Could you check a few things on this model? Use its own coordinates, in mm. Face numbers are marked on the shaded views. Coordinates: 2 decimals unless noted, no trailing zeros. Loops run counter-clockwise (first coordinate to the right, second up) from the corner with the lowest first, then second, coordinate; pieces in that order, holes last.
from build123d import *

# Parameters (mm, degrees)
GEARBOX_MOUNT_DEPTH  = 77
BOSS_EXTRUDE6_START  = 38
SKETCH7_R            = 1.7
SKETCH7_W            = 1
SKETCH7_H            = 6
BOSS_EXTRUDE6_DEPTH  = 1
BOSS_EXTRUDE7_START  = 76
SKETCH8_R            = 1.25
SKETCH8_R_2          = 1.7
SKETCH8_W            = 1
SKETCH8_H            = 6
BOSS_EXTRUDE7_DEPTH  = 1
CUT_EXTRUDE1_START   = 22.5
CUT_EXTRUDE1_DEPTH   = 8
BOSS_EXTRUDE9_START  = 22.5
BOSS_EXTRUDE9_DEPTH  = 2
SKETCH12_W           = 10.2
SKETCH12_H           = 12
SKETCH12_R           = 1.7
BOSS_EXTRUDE10_DEPTH = 2
CUT_EXTRUDE2_START   = 24.5
SKETCH9_W            = 7
SKETCH9_H            = 1
CUT_EXTRUDE2_DEPTH   = 6
CUT_EXTRUDE3_START   = 39
CUT_EXTRUDE3_DEPTH   = 36


with BuildPart() as part:
    # Sketch2 → Gearbox Mount (new body)
    with BuildSketch(Plane.XY):
        Polygon((-24.506477671, 70.636122542), (-24.506477671, 76.636122542), (-25.506477671, 76.636122542), (-25.506477671, 70.636122542), (-35.706477671, 70.636122542), (-35.706477671, 76.636122542), (-37.706477671, 76.636122542), (-37.706477671, 69.636122542), (-12.306477671, 69.636122542), (-12.306477671, 76.636122542), (-14.306477671, 76.636122542), (-14.306477671, 70.636122542), align=None)
    extrude(amount=GEARBOX_MOUNT_DEPTH)

    # Sketch7 → Boss-Extrude6 (add, symmetric)
    with BuildSketch(Plane.XY.offset(BOSS_EXTRUDE6_START)):
        Polygon((-24.506477671, 76.636122542), (-24.506477671, 70.636122542), (-14.306477671, 70.636122542), (-14.306477671, 76.636122542), (-14.306477671, 82.636122542), (-24.506477671, 82.636122542), align=None)
        with Locations((-19.406477671, 76.636122542)):
            Circle(SKETCH7_R, mode=Mode.SUBTRACT)
        with Locations((-25.006477671, 79.636122542)):
            Rectangle(SKETCH7_W, SKETCH7_H)
        Polygon((-25.506477671, 70.636122542), (-25.506477671, 76.636122542), (-25.506477671, 82.636122542), (-35.706477671, 82.636122542), (-35.706477671, 70.636122542), align=None)
        with Locations((-30.606477671, 76.636122542)):
            Circle(SKETCH7_R, mode=Mode.SUBTRACT)
    extrude(amount=BOSS_EXTRUDE6_DEPTH, both=True)

    # Sketch8 → Boss-Extrude7 (add, symmetric)
    with BuildSketch(Plane.XY.offset(BOSS_EXTRUDE7_START)):
        Polygon((-35.706477671, 82.636122542), (-35.706477671, 70.636122542), (-25.506477671, 70.636122542), (-25.506477671, 76.636122542), (-25.506477671, 82.636122542), align=None)
        with Locations((-30.606477671, 72.786122542)):
            Circle(SKETCH8_R, mode=Mode.SUBTRACT)
        with Locations((-30.606477671, 76.636122542)):
            Circle(SKETCH8_R_2, mode=Mode.SUBTRACT)
        with Locations((-25.006477671, 79.636122542)):
            Rectangle(SKETCH8_W, SKETCH8_H)
        Polygon((-14.306477671, 82.636122542), (-24.506477671, 82.636122542), (-24.506477671, 76.636122542), (-24.506477671, 70.636122542), (-14.306477671, 70.636122542), (-14.306477671, 76.636122542), align=None)
        with Locations((-19.406477671, 72.786122542)):
            Circle(SKETCH8_R, mode=Mode.SUBTRACT)
        with Locations((-19.406477671, 76.636122542)):
            Circle(SKETCH8_R_2, mode=Mode.SUBTRACT)
    extrude(amount=BOSS_EXTRUDE7_DEPTH, both=True)

    # Sketch10 → Cut-Extrude1 (cut)
    with BuildSketch(Plane.XY.offset(CUT_EXTRUDE1_START)):
        Polygon((-14.306477671, 70.636122542), (-14.306477671, 72.136122542), (-12.306477671, 72.136122542), (-12.306477671, 82.636122542), (-37.706477671, 82.636122542), (-37.706477671, 72.136122542), (-35.706477671, 72.136122542), (-35.706477671, 70.636122542), (-25.506477671, 70.636122542), (-25.506477671, 72.136122542), (-24.506477671, 72.136122542), (-24.506477671, 70.636122542), align=None)
    extrude(amount=CUT_EXTRUDE1_DEPTH, mode=Mode.SUBTRACT)

    # Sketch11 → Boss-Extrude9 (add)
    with BuildSketch(Plane.XY.offset(BOSS_EXTRUDE9_START)):
        with BuildLine():
            Line((-24.506477671, 76.636122542), (-24.506477671, 70.636122542))
            Line((-24.506477671, 70.636122542), (-14.306477671, 70.636122542))
            Line((-14.306477671, 70.636122542), (-14.306477671, 76.636122542))
            Line((-14.306477671, 76.636122542), (-17.706477671, 76.636122542))
            ThreePointArc((-17.706477671, 76.636122542), (-19.406477671, 74.936122542), (-21.106477671, 76.636122542))
            Line((-21.106477671, 76.636122542), (-24.506477671, 76.636122542))
        make_face()
    extrude(amount=-BOSS_EXTRUDE9_DEPTH)

    # Sketch12 → Boss-Extrude10 (add)
    with BuildSketch(Plane.XY):
        with Locations((-19.406477671, 76.636122542)):
            Rectangle(SKETCH12_W, SKETCH12_H)
        with Locations((-19.406477671, 76.636122542)):
            Circle(SKETCH12_R, mode=Mode.SUBTRACT)
    extrude(amount=BOSS_EXTRUDE10_DEPTH)

    # Sketch9 → Cut-Extrude2 (cut)
    with BuildSketch(Plane.XY.offset(CUT_EXTRUDE2_START)):
        with Locations((-30.606477671, 70.136122542)):
            Rectangle(SKETCH9_W, SKETCH9_H)
        with Locations((-19.406477671, 70.136122542)):
            Rectangle(SKETCH9_W, SKETCH9_H)
    extrude(amount=CUT_EXTRUDE2_DEPTH, mode=Mode.SUBTRACT)

    # Sketch13 → Cut-Extrude3 (cut)
    with BuildSketch(Plane.XY.offset(CUT_EXTRUDE3_START)):
        Polygon((-19.406477671, 69.636122542), (-21.406477671, 69.636122542), (-21.406477671, 70.636122542), (-17.406477671, 70.636122542), (-17.406477671, 69.636122542), align=None)
        Polygon((-30.606477671, 69.636122542), (-32.606477671, 69.636122542), (-32.606477671, 70.636122542), (-28.606477671, 70.636122542), (-28.606477671, 69.636122542), align=None)
    extrude(amount=CUT_EXTRUDE3_DEPTH, mode=Mode.SUBTRACT)


solid = part.part
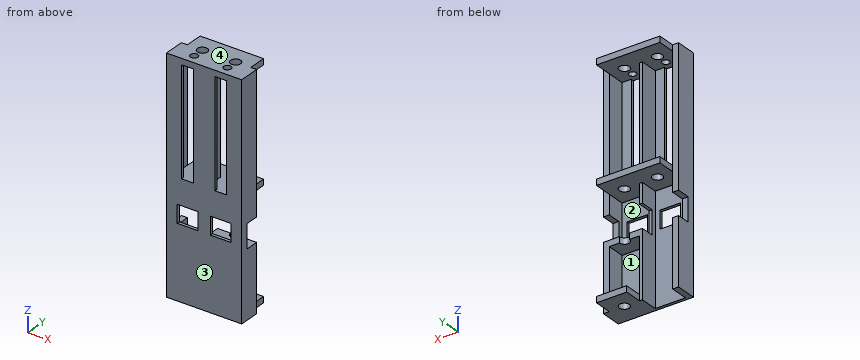
(1) Imagine slicing it at B-B, the plane z = 57.5. Write out the boundary of the cut face in (x, y).
Answers:
outline: (-37.71, 69.64) - (-32.61, 69.64) - (-32.61, 70.64) - (-35.71, 70.64) - (-35.71, 76.64) - (-37.71, 76.64) - close; (-28.61, 69.64) - (-21.41, 69.64) - (-21.41, 70.64) - (-24.51, 70.64) - (-24.51, 76.64) - (-25.51, 76.64) - (-25.51, 70.64) - (-28.61, 70.64) - close; (-17.41, 69.64) - (-12.31, 69.64) - (-12.31, 76.64) - (-14.31, 76.64) - (-14.31, 70.64) - (-17.41, 70.64) - close
(2) Imagine slicing it at C-C, the plane z = 16.5. Write out the boundary of the cut face in (x, y).
Answers:
outline: (-37.71, 69.64) - (-12.31, 69.64) - (-12.31, 76.64) - (-14.31, 76.64) - (-14.31, 70.64) - (-24.51, 70.64) - (-24.51, 76.64) - (-25.51, 76.64) - (-25.51, 70.64) - (-35.71, 70.64) - (-35.71, 76.64) - (-37.71, 76.64) - close
(3) Imagine slicing it at A-A, the plane y = 81. Write out the boundary of the cut face in (x, z).
Answers:
outline: (-35.71, 37) - (-14.31, 37) - (-14.31, 39) - (-35.71, 39) - close; (-35.71, 75) - (-14.31, 75) - (-14.31, 77) - (-35.71, 77) - close; (-24.51, 0) - (-14.31, 0) - (-14.31, 2) - (-24.51, 2) - close
(4) We'd pull the mould along Z, two halves only. Please class the marked faces 1, 2, 3 and 4: +Z half, -Z half, draft (parallel to the pull), parting line (faces both ways), or undercut.
Answers:
face 1: undercut
face 2: undercut
face 3: draft
face 4: +Z half
(5) For pin 1 (2.5 mm diameter, centred on x = -26.5, z = 58, fed in from +Y); pin 2 (0.6 mm diameter, centred on x = -37, z = 27.5, fed in from +Y); pin 3 (1 mm diameter, centred on x = -31, y = 80, fed in from -Z), each with a flat end and sliding along its axis, tell me the tip position at first contact or that it passes through.
Answers:
pin 1: stops at y = 76.64
pin 2: stops at y = 72.14
pin 3: stops at z = 37
(6) I need wall thicknesses on probe 1 along X at (y, z) = (73.75, 18.5); probe 2 along Z at (x, y) = (-14.5, 79.5); probe 3 along Z at (x, y) = (-22, 70.75). Which ranges of each line are inside material? Lowest first, please.
Answers:
probe 1: x = -37.71 to -35.71, -25.51 to -24.51, -14.31 to -12.31
probe 2: z = 0 to 2, 37 to 39, 75 to 77
probe 3: z = 0 to 2, 20.5 to 22.5, 37 to 39, 75 to 77
